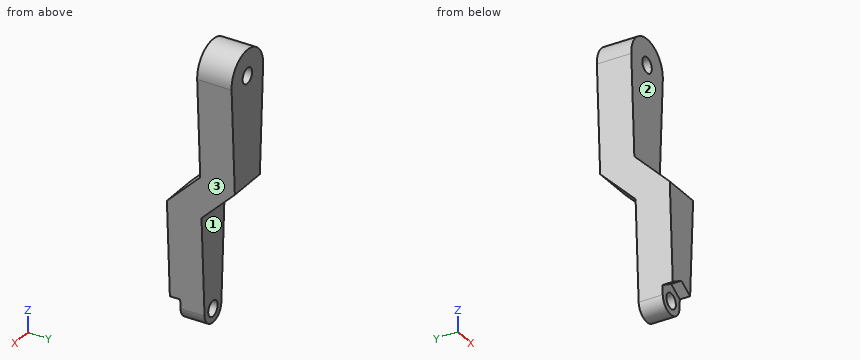
from build123d import *

# Parameters (mm, degrees)
SKETCH1_R           = 1.125
BOSS_EXTRUDE1_DEPTH = 10
CUT_EXTRUDE1_START  = -5
SKETCH2_R           = 1.125
CUT_EXTRUDE1_DEPTH  = 5
CUT_EXTRUDE3_START  = -10
SKETCH2_4_R         = 1.125
CUT_EXTRUDE3_DEPTH  = 5
CHAMFER1_SIZE       = 5
CUT_EXTRUDE4_DEPTH  = 1.5


with BuildPart() as part:
    # Sketch1 → Boss-Extrude1 (new body)
    with BuildSketch(Plane(origin=(0, 0, 0), x_dir=(1, 0, 0), z_dir=(0, 1, 0))):
        with BuildLine():
            ThreePointArc((-3.745309567, 0.1875), (0, -3.75), (3.745309567, 0.1875))
            Line((3.745309567, 0.1875), (1.997498436, 35.1))
            ThreePointArc((1.997498436, 35.1), (0, 37), (-1.997498436, 35.1))
            Line((-1.997498436, 35.1), (-3.745309567, 0.1875))
        make_face()
        with Locations(Location((0, 0, 0), (0, 0, 270))):
            Circle(SKETCH1_R, mode=Mode.SUBTRACT)
        with Locations(Location((0, 35, 0), (0, 0, 270))):
            Circle(SKETCH1_R, mode=Mode.SUBTRACT)
    extrude(amount=BOSS_EXTRUDE1_DEPTH)

    # Sketch2 → Cut-Extrude1 (cut)
    with BuildSketch(Plane(origin=(0, 10, 0), x_dir=(1, 0, 0), z_dir=(0, 1, 0)).offset(CUT_EXTRUDE1_START)):
        with BuildLine():
            Line((-1.997498436, 35.1), (-2.721216149, 20.64375))
            Line((-2.721216149, 20.64375), (2.721216149, 20.64375))
            Line((2.721216149, 20.64375), (1.997498436, 35.1))
            ThreePointArc((1.997498436, 35.1), (0, 37), (-1.997498436, 35.1))
        make_face()
        with Locations(Location((0, 35, 0), (0, 0, 270))):
            Circle(SKETCH2_R, mode=Mode.SUBTRACT)
    extrude(amount=CUT_EXTRUDE1_DEPTH, mode=Mode.SUBTRACT)

    # Sketch2<4> → Cut-Extrude3 (cut)
    # profile 1 of 2: a face of its own
    with BuildSketch(Plane(origin=(0, 10, 0), x_dir=(1, 0, 0), z_dir=(0, 1, 0)).offset(CUT_EXTRUDE3_START)):
        with BuildLine():
            ThreePointArc((3.745309567, 0.1875), (0, 3.75), (-3.745309567, 0.1875))
            ThreePointArc((-3.745309567, 0.1875), (-0.093779329, -3.748827208), (3.75, 0))
            ThreePointArc((3.75, 0), (3.748827208, 0.093779329), (3.745309567, 0.1875))
        make_face()
        with Locations(Location((0, 0, 0), (0, 0, 270))):
            Circle(SKETCH2_4_R, mode=Mode.SUBTRACT)
    # profile 2 of 2: a face of its own
    with BuildSketch(Plane(origin=(0, 10, 0), x_dir=(1, 0, 0), z_dir=(0, 1, 0)).offset(CUT_EXTRUDE3_START)):
        with BuildLine():
            Line((3.021591853, 14.64375), (-3.021591853, 14.64375))
            Line((-3.021591853, 14.64375), (-3.745309567, 0.1875))
            ThreePointArc((-3.745309567, 0.1875), (0, 3.75), (3.745309567, 0.1875))
            Line((3.745309567, 0.1875), (3.021591853, 14.64375))
        make_face()
    extrude(amount=CUT_EXTRUDE3_DEPTH, mode=Mode.SUBTRACT)

    # Chamfer1
    chamfer1_edges = [part.edges().sort_by_distance(p)[0] for p in [
        (0, 0, -14.64375),
        (0, 10, -20.64375),
    ]]
    chamfer(chamfer1_edges, length=CHAMFER1_SIZE - 0.0001)  # a hair under: the kernel refuses the full size

    # Sketch3 → Cut-Extrude4 (cut)
    with BuildSketch(Plane.XZ):
        Polygon((0, -32.546261356), (-2.125, -33.773130678), (-2.125, -36.226869322), (0, -37.453738644), (2.125, -36.226869322), (2.125, -33.773130678), align=None)
    extrude(amount=-CUT_EXTRUDE4_DEPTH, mode=Mode.SUBTRACT)


solid = part.part
Design review of the part built by this model. Coordinates are the model's own, in mm. Face numbers are marked on the shaded views. A direction names the side the tool comes from. Round coordinates to 2 decimals unless told otherwise and drop trailing zeros. Loops run counter-clockwise (first coordinate to the right, second up) from the corner with the lowest first, then second, coordinate; pieces in that order, holes last. Notation, with made-up numbers: (35.25, 79) - (81.25, 79) arc R18 ccw to (81.25, 97) - close; hole circle Ø7 at (27.5, 61). An arc over 180 degrees is marked (long way). One line per item, written item: value. Start each with the question number.
1) Insertion check: pin 1 Ø3 at (x, z) = (1.5, -17.5) entering from -Y; pin 2 Ø4.5 at (x, z) = (-0.5, -33) entering from +Y; pin 3 Ø4 at (x, z) = (0, -2) entering from -Y; pin 4 Ø4 at (x, y) = (-1, 6.5) entering from +Z. Each pin has a flat end and moves straight along its axis. Give the tip position at first contact, or say it passes through.
2) For the marked faces 1, 2 and 3, list the 3-axis set-ups (+Z, -Z, +X, -X, +Y, -Y) from which the entire face can be reached by the end or side of a thin tool; tool diameter is ignored.
3) Consider section D-D on z = -3.5. Give the boundary of the cut face in (x, y).
4) Consider section C-C on z = -9.5. Give the boundary of the cut face in (x, y), then the cut area to 3 significant figures.
5) To check wall thickness, follow L1, parallel to X at y = 2.3, z = -35 (1 decimal); L2, parallel to X at y = 6.2, z = 0 (3 decimals); L3, parallel to Y at x = -1.5, z = -23. State the ranges of each line that lie inside material, in increasing order. Write a range as from..to.
6) Consider section A-A on x = 0.5. Give the number of separate pieces and of enclosed holes in the cut face, then the cut area to 3 significant figures.
Reported:
1. pin 1: stops at y = 0.64
1. pin 2: stops at y = 5
1. pin 3: stops at y = 5
1. pin 4: stops at z = 3.75
2. face 1: -Z, +X, -X, +Y
2. face 2: +Z, +X, -X, -Y
2. face 3: -Z, +X, +Y, -Y
3. outline: (-3.58, 5) - (3.58, 5) - (3.58, 10) - (-3.58, 10) - close
4. outline: (-3.28, 5) - (3.28, 5) - (3.28, 10) - (-3.28, 10) - close
4. area: 32.8 mm^2
5. L1: x = -2..-1.1, 1.1..2
5. L2: x = -3.75..-1.125, 1.125..3.75
5. L3: y = 0..5
6. separate pieces: 3
6. enclosed holes: 0
6. area: 185 mm^2
